```python
from build123d import *

# Parameters (mm, degrees)
F0_W      = 121.92
F0_H      = 98.552
F1_DEPTH  = 3.175
F2_W      = 12.7
F2_H      = 3.175
F3_DEPTH  = 6.35
F4_W      = 12.7
F4_H      = 3.175
F5_DEPTH  = 6.35
F6_R      = 6.34999
F7_R      = 1.905
F8_DEPTH  = 6.35
F9_W      = 115.57
F9_H      = 3.175
F10_DEPTH = 31.75
F11_R     = 2.921
F11_R_2   = 1.016
F12_R     = 2.794
F12_R_2   = 1.016
F13_R     = 2.921
F13_R_2   = 1.016
F14_DEPTH = 5.08


# Not quite as in the source:
# - a fillet or chamfer is up to 0.001 mm smaller than in the source, because OpenCascade refuses the exact size
# - a feature names something its author has since deleted; it is built from what else it names


with BuildPart() as f1:
    # F0 (on Top) → F1 (new body)
    with BuildSketch(Plane.XY):
        with Locations((-12.7, -8.001)):
            Rectangle(F0_W, F0_H)
    extrude(amount=F1_DEPTH)

    # F2 (on face) → F3 (join)
    with BuildSketch(Plane.YZ.offset(48.26)):
        with Locations((-19.177, 1.5875)):
            Rectangle(F2_W, F2_H)
    extrude(amount=F3_DEPTH)

    # F4 (on face) → F5 (join)
    with BuildSketch(Plane(origin=(-73.66, 0, 0), x_dir=(0, -1, 0), z_dir=(-1, 0, 0))):
        with Locations((19.177, 1.5875)):
            Rectangle(F4_W, F4_H)
    extrude(amount=F5_DEPTH)

    # F6 (radius 6.35 in the source; OpenCascade refuses exactly that, so slightly less here)
    f6_edges = [f1.edges().sort_by_distance(p)[0] for p in [
        (-80.01, -25.527, 1.5875),
        (-80.01, -12.827, 1.5875),
        (54.61, -25.527, 1.5875),
        (54.61, -12.827, 1.5875),
    ]]
    fillet(f6_edges, radius=F6_R)

    # F7 (on face) → F8 (cut)
    with BuildSketch(Plane.XY.offset(3.175)):
        with Locations((-76.835, -19.177)):
            Circle(F7_R)
        with Locations((51.435, -19.177)):
            Circle(F7_R)
    extrude(amount=-F8_DEPTH, mode=Mode.SUBTRACT)

    # F9 (on face) → F10 (join)
    with BuildSketch(Plane.XY.offset(3.175)):
        Polygon((-73.66, -57.277), (-70.485, -57.277), (-70.485, -54.102), (-70.485, 38.1), (-70.485, 41.275), (-73.66, 41.275), (-73.66, -12.827), (-73.66, -25.527), align=None)
        with Locations((-12.7, -55.6895)):
            Rectangle(F9_W, F9_H)
        with Locations((-12.7, 39.6875)):
            Rectangle(F9_W, F9_H)
        Polygon((45.085, -57.277), (48.26, -57.277), (48.26, -25.527), (48.26, -12.827), (48.26, 41.275), (45.085, 41.275), (45.085, 38.1), (45.085, -54.102), align=None)
    extrude(amount=F10_DEPTH)

    # F11 (on face) + F12 (on face) + F13 (on face) → F14 (join)
    with BuildSketch(Plane.XY.offset(3.175)):
        with Locations((-63.754, 30.607)):
            Circle(F11_R)
        with Locations((-63.754, 30.607)):
            Circle(F11_R_2, mode=Mode.SUBTRACT)
        with Locations((-14.732, -27.559)):
            Circle(F11_R)
        with Locations((-14.732, -27.559)):
            Circle(F11_R_2, mode=Mode.SUBTRACT)
        with Locations((-14.732, 30.607)):
            Circle(F11_R)
        with Locations((-14.732, 30.607)):
            Circle(F11_R_2, mode=Mode.SUBTRACT)
        with Locations((-63.754, -27.559)):
            Circle(F11_R)
        with Locations((-63.754, -27.559)):
            Circle(F11_R_2, mode=Mode.SUBTRACT)
    with BuildSketch(Plane.XY.offset(3.175)):
        with Locations((34.798, 14.605)):
            Circle(F12_R)
        with Locations((34.798, 14.605)):
            Circle(F12_R_2, mode=Mode.SUBTRACT)
        with Locations((0.762, 32.131)):
            Circle(F12_R)
        with Locations((0.762, 32.131)):
            Circle(F12_R_2, mode=Mode.SUBTRACT)
    with BuildSketch(Plane.XY.offset(3.175)):
        with Locations((40.005, -19.05)):
            Circle(F13_R)
        with Locations((40.005, -19.05)):
            Circle(F13_R_2, mode=Mode.SUBTRACT)
        with Locations((40.005, -49.022)):
            Circle(F13_R)
        with Locations((40.005, -49.022)):
            Circle(F13_R_2, mode=Mode.SUBTRACT)
        with Locations((-0.127, -49.022)):
            Circle(F13_R)
        with Locations((-0.127, -49.022)):
            Circle(F13_R_2, mode=Mode.SUBTRACT)
        with Locations((-0.127, -19.05)):
            Circle(F13_R)
        with Locations((-0.127, -19.05)):
            Circle(F13_R_2, mode=Mode.SUBTRACT)
    extrude(amount=F14_DEPTH)


solid = f1.part
```
The model under review builds one solid part; all positions refer to its coordinate system, in mm. A direction names the side the tool comes from. Round coordinates to 2 decimals unless told otherwise and drop trailing zeros. Write each loop counter-clockwise with the first axis right and the second up, starting at its lowest first coordinate (ties: lowest second). Pieces come first, ordered by that corner, then holes. Notation, with made-up numbers: M 17.5,53.25 L 57.5,53.25 A18 ccw 57.5,61.25 Z; hole C 15,10.5 d11. An arc over 180 degrees is marked long. Use CSV: the item, a comma, the result in double quotes. Start each with the question number.
(1) Tool access review of faces 1 (the face through (49, -19, 3.175)), 2 (the face through (-74.76, -19.09, 3.175)), 3 (the face through (52.8, -14.74, 1.61)), 4 (the face through (-0.2, -50.3, 8.255)): name each direction out of +Z, -Z, +X, -X, +Y, -Y from which nothing blocks a thin tool from reaching the whole face with its end or side.
(2) For line 1 along X through (y, z) = (-9, 23) (3 decimals); line 2 along Y through (x, z) = (32.5, 32.5) (3 decimals); line 3 along Z through (x, y) = (-46.5, 28) (3 decimals), list the stretches that pass through material, from the lowest coordinate up.
(3) We need section A-A, the plane z = 29. State the section outline as (x, y) points (3 decimals), then the cut area to 3 significant figures.
(4) We need section B-B, the plane y = 20. State the section outline as (x, z) points (3 decimals).
(5) Clearance check with flat-ended pins moving along their axes: P1, Ø1.8, axis at x = 40.005, y = -49.022, coming from the +Z side (3 decimals); P2, Ø8, axis at y = 0, z = 7.5, coming from the +X side; P3, Ø4.5, axis at x = -1.5, y = -48.5, coming from the +Z side (3 decimals). State where each tip first meets the part, or that it passes through.
(6) We need section C-C, the plane x = 26. State the section outline as (y, z) points (3 decimals).
(7) The part is to be moulded in two halves that separate along X. For faces 5 (the face through (-78.1, -23.716, 1.61)), 6 (the face through (-0.507, -46.126, 5.679)), 7 (the face through (-70.485, -9, 19)), 8 (the face through (-14, -7, 0)), say which applies: +X half, -X half, draft (parallel to the pull), parting line (faces both ways), or undercut.
Findings:
1,face 1,"+Z, +X, +Y, -Y"
1,face 2,"+Z, -X, +Y, -Y"
1,face 3,"+Z, -Z, +X, +Y"
1,face 4,"+Z"
2,line 1,"-73.66 to -70.485, 45.085 to 48.26"
2,line 2,"-57.277 to -54.102, 38.1 to 41.275"
2,line 3,"0 to 3.175"
3,outline,"M -73.66,-57.277 L 48.26,-57.277 L 48.26,41.275 L -73.66,41.275 Z; hole M -70.485,-54.102 L 45.085,-54.102 L 45.085,38.1 L -70.485,38.1 Z"
3,area,"1,360 mm^2"
4,outline,"M -73.66,0 L 48.26,0 L 48.26,34.925 L 45.085,34.925 L 45.085,3.175 L -70.485,3.175 L -70.485,34.925 L -73.66,34.925 Z"
5,P1,"z = 3.175"
5,P2,"x = 48.26"
5,P3,"z = 8.255"
6,outline,"M -57.277,0 L 41.275,0 L 41.275,34.925 L 38.1,34.925 L 38.1,3.175 L -54.102,3.175 L -54.102,34.925 L -57.277,34.925 Z"
7,face 5,"-X half"
7,face 6,"undercut"
7,face 7,"undercut"
7,face 8,"draft"
